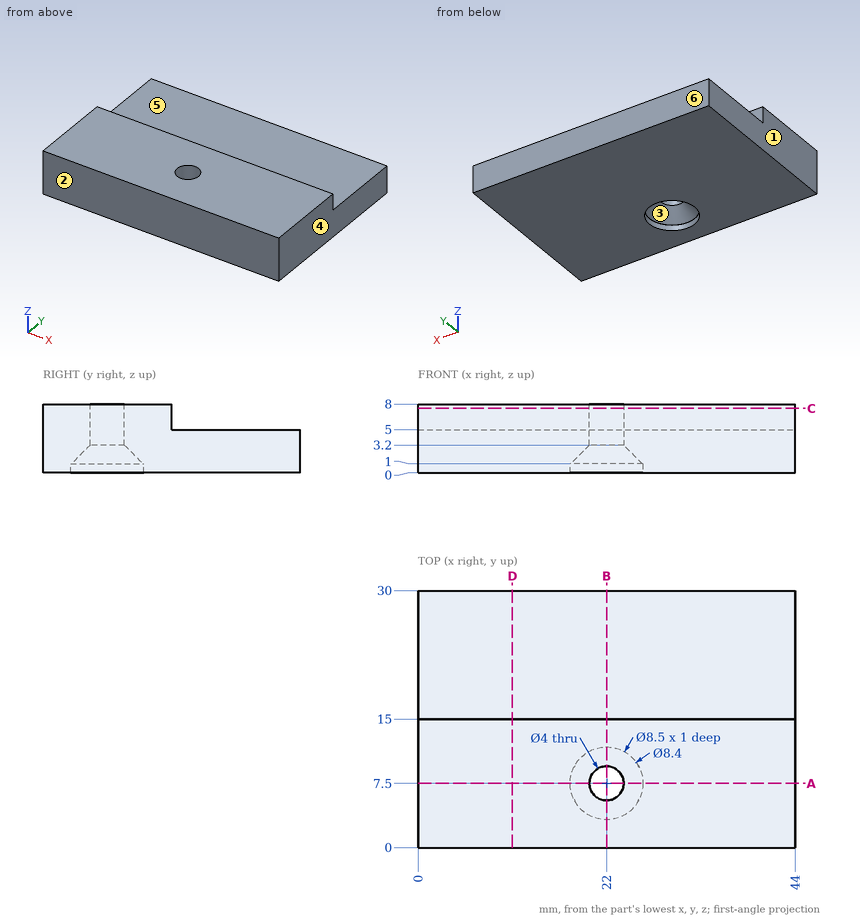
Part print with two shaded views. Sizes in mm from the minimum x, y, z corner. A direction names the side the tool comes from. Round coordinates to 2 decimals unless told otherwise and drop trailing zeros. Order: outer loops, then holes, each group sorted by start corner. A loop starts at its lowest first (then second) coordinate and runs counter-clockwise, first axis right, second up. Notation, with made-up numbers: (-27, 10.25) - (19, 10.25) arc R27 ccw to (19, 40.25) - close; hole circle Ø10 at (3.5, -27). An arc over 180 degrees is marked (long way). Answer in a Markdown table with one row per item. Add a question column.
(1) Band-saw the part on A-A on y = 7.5. List the corners of the cut face in (x, z).
(2) Mould opens along X. For the marked faces 1, 2, 3 and 4 say: +X half, -X half, draft (parallel to the pull), parting line (faces both ways), or undercut.
(3) Probe L1, parallel to Y at x = 22, z = 0.35; L2, parallel to Y at x = 22, z = 5.15; L3, parallel to X at y = 7.5, z = 5.1. List the from-to ranges inside material, lowest first. Write a range as [from, to].
(4) Band-saw the part on D-D on x = 11. List the corners of the cut face in (y, z), and give its area (3 significant figures).
(5) Band-saw the part on C-C on z = 7.5. List the corners of the cut face in (x, y).
(6) Drop flat-ended pins along their axis: pin 1 Ø2.5 at (x, y) = (20.5, 9.5) entering from -Z; pin 2 Ø2.5 at (x, z) = (24, 6.5) entering from +Y; pin 3 Ø5 at (x, y) = (22, 7.5) entering from -Z. Give the stop position or say it passes through.
(7) 3-axis set-ups, long thin cutter, end or side, ignore diameter. For the marked faces 5 and 6: which of +Z, -Z, +X, -X, +Y, -Y reach the whole face in a straight line?
(8) Band-saw the part on B-B on x = 22. List the corners of the cut face in (y, z), and give its area (3 significant figures).
Data:
| question | item | result |
|---|---|---|
| 1 | outline | (0, 0) - (17.75, 0) - (17.75, 1) - (17.8, 1) - (20, 3.2) - (20, 8) - (0, 8) - close; (24, 3.2) - (26.2, 1) - (26.25, 1) - (26.25, 0) - (44, 0) - (44, 8) - (24, 8) - close |
| 2 | face 1 | -X half |
| 2 | face 2 | draft |
| 2 | face 3 | undercut |
| 2 | face 4 | +X half |
| 3 | L1 | y = [0, 3.25], [11.75, 30] |
| 3 | L2 | y = [0, 5.5], [9.5, 15] |
| 3 | L3 | x = [0, 20], [24, 44] |
| 4 | outline | (0, 0) - (30, 0) - (30, 5) - (15, 5) - (15, 8) - (0, 8) - close |
| 4 | area | 195 mm^2 |
| 5 | outline | (0, 0) - (44, 0) - (44, 15) - (0, 15) - close; hole circle Ø4 at (22, 7.5) |
| 6 | pin 1 | stops at z = 1.45 |
| 6 | pin 2 | stops at y = 15 |
| 6 | pin 3 | stops at z = 2.7 |
| 7 | face 5 | +Z, +X, -X, +Y |
| 7 | face 6 | +Z, -Z, +X, -X, +Y |
| 8 | outline | (0, 0) - (3.25, 0) - (3.25, 1) - (3.3, 1) - (5.5, 3.2) - (5.5, 8) - (0, 8) - close; (9.5, 3.2) - (11.7, 1) - (11.75, 1) - (11.75, 0) - (30, 0) - (30, 5) - (15, 5) - (15, 8) - (9.5, 8) - close |
| 8 | area | 154 mm^2 |
